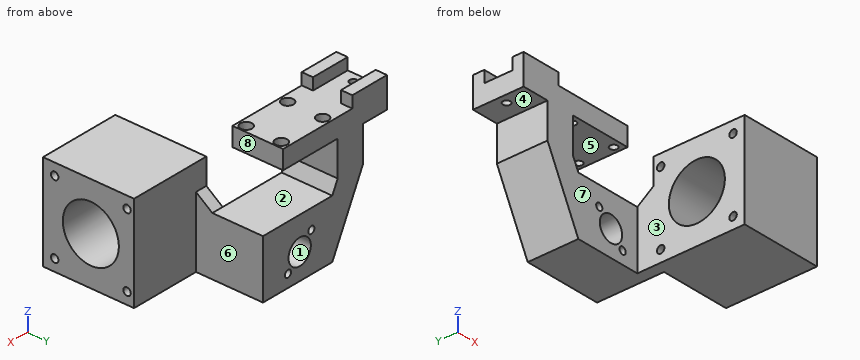
```python
from build123d import *

# Parameters (mm, degrees)
SKICA1_W                 = 50.278910674
SKICA1_H                 = 21.7
SKICA1_R                 = 1.6
P_IDAT_VYSUNUT_M1_DEPTH  = 8
SKICA2_R                 = 2.5
ODEBRAT_VYSUNUT_M1_DEPTH = 4
SKICA3_R                 = 1.6
ODEBRAT_VYSUNUT_M2_DEPTH = 8
SKICA4_W                 = 12.327690559
SKICA4_H                 = 21.7
P_IDAT_VYSUNUT_M2_DEPTH  = 15
SKICA6_R                 = 5.406276896
P_IDAT_VYSUNUT_M3_DEPTH  = 21.7
SKICA7_R                 = 1.5
ODEBRAT_VYSUNUT_M3_DEPTH = 21.7
SKICA9_R                 = 1.6
SKICA9_R_2               = 12
P_IDAT_VYSUNUT_M4_DEPTH  = 5
SKICA10_W                = 41
SKICA10_H                = 39
SKICA10_R                = 12
SKICA10_R_2              = 1.6
P_IDAT_VYSUNUT_M5_DEPTH  = 30
SKICA11_W                = 16.773929501
SKICA11_H                = 4.85
P_IDAT_VYSUNUT_M6_DEPTH  = 5


with BuildPart() as part:
    # Skica1 → Přidat vysunutím1 (new body)
    with BuildSketch(Plane.XY):
        with Locations((-8.927473885, -9.09140889)):
            Rectangle(SKICA1_W, SKICA1_H)
        with Locations((13.311981452, -16.59140889)):
            Circle(SKICA1_R, mode=Mode.SUBTRACT)
        with Locations((-6.688018548, -16.59140889)):
            Circle(SKICA1_R, mode=Mode.SUBTRACT)
        with Locations((-6.688018548, -1.59140889)):
            Circle(SKICA1_R, mode=Mode.SUBTRACT)
        with Locations((13.311981452, -1.59140889)):
            Circle(SKICA1_R, mode=Mode.SUBTRACT)
    extrude(amount=P_IDAT_VYSUNUT_M1_DEPTH)

    # Skica2 → Odebrat vysunutím1 (cut)
    with BuildSketch(Plane.XY.offset(8)):
        with Locations((13.311981452, -16.59140889)):
            Circle(SKICA2_R)
        with Locations((-6.688018548, -16.59140889)):
            Circle(SKICA2_R)
        with Locations((-6.688018548, -1.59140889)):
            Circle(SKICA2_R)
        with Locations((13.311981452, -1.59140889)):
            Circle(SKICA2_R)
    extrude(amount=-ODEBRAT_VYSUNUT_M1_DEPTH, mode=Mode.SUBTRACT)

    # Skica3 → Odebrat vysunutím2 (cut)
    with BuildSketch(Plane.XY.offset(8)):
        with Locations((-30.066929222, -9.09140889)):
            Circle(SKICA3_R)
    extrude(amount=-ODEBRAT_VYSUNUT_M2_DEPTH, mode=Mode.SUBTRACT)

    # Skica4 → Přidat vysunutím2 (add)
    with BuildSketch(Plane(origin=(0, 0, 0), x_dir=(-1, 0, 0), z_dir=(0, 0, -1))):
        with Locations((16.351863828, -9.09140889)):
            Rectangle(SKICA4_W, SKICA4_H)
    extrude(amount=P_IDAT_VYSUNUT_M2_DEPTH)

    # Skica6 → Přidat vysunutím3 (add)
    with BuildSketch(Plane(origin=(0, 1.75859111, 0), x_dir=(1, 0, 0), z_dir=(0, 1, 0))):
        Polygon((-22.515709107, 15), (-10.188018548, 15), (-7.585826442, 20.254970434), (20.97371307, 20.254970434), (20.97371307, 45.15), (4.741864117, 45.15), (-7.585826442, 45.15), align=None)
        with Locations(Location((8.208247023, 34.15, 0), (0, 0, 270))):
            Circle(SKICA6_R, mode=Mode.SUBTRACT)
    extrude(amount=-P_IDAT_VYSUNUT_M3_DEPTH)

    # Skica7 → Odebrat vysunutím3 (cut)
    with BuildSketch(Plane.XZ.offset(19.94140889)):
        with Locations(Location((2.551392773, -28.493145751, 0), (0, 0, 270))):
            Circle(SKICA7_R)
        with Locations(Location((13.865101272, -39.806854249, 0), (0, 0, 270))):
            Circle(SKICA7_R)
    extrude(amount=-ODEBRAT_VYSUNUT_M3_DEPTH, mode=Mode.SUBTRACT)

    # Skica9 → Přidat vysunutím4 (add)
    with BuildSketch(Plane(origin=(20.97371307, 0, 0), x_dir=(0, 0, -1), z_dir=(1, 0, 0))):
        Polygon((45.15, 1.75859111), (20.254970434, 1.75859111), (20.254970434, -19.94140889), (15.15, -26.94140889), (4.15, -26.94140889), (4.15, -65.94140889), (15.15, -65.94140889), (45.15, -65.94140889), (45.15, -19.94140889), align=None)
        with Locations((40.15, -60.94140889)):
            Circle(SKICA9_R, mode=Mode.SUBTRACT)
        with Locations((9.15, -60.94140889)):
            Circle(SKICA9_R, mode=Mode.SUBTRACT)
        with Locations((9.15, -29.94140889)):
            Circle(SKICA9_R, mode=Mode.SUBTRACT)
        with Locations((40.15, -29.94140889)):
            Circle(SKICA9_R, mode=Mode.SUBTRACT)
        with Locations((24.65, -45.44140889)):
            Circle(SKICA9_R_2, mode=Mode.SUBTRACT)
    extrude(amount=P_IDAT_VYSUNUT_M4_DEPTH)

    # Skica10 → Přidat vysunutím5 (add)
    with BuildSketch(Plane(origin=(25.97371307, 0, 0), x_dir=(0, 0, -1), z_dir=(1, 0, 0))):
        with Locations((24.65, -46.44140889)):
            Rectangle(SKICA10_W, SKICA10_H)
        with Locations((24.65, -45.44140889)):
            Circle(SKICA10_R, mode=Mode.SUBTRACT)
        with Locations((40.15, -60.94140889)):
            Circle(SKICA10_R_2, mode=Mode.SUBTRACT)
        with Locations((40.15, -29.94140889)):
            Circle(SKICA10_R_2, mode=Mode.SUBTRACT)
        with Locations((9.15, -29.94140889)):
            Circle(SKICA10_R_2, mode=Mode.SUBTRACT)
        with Locations((9.15, -60.94140889)):
            Circle(SKICA10_R_2, mode=Mode.SUBTRACT)
    extrude(amount=P_IDAT_VYSUNUT_M5_DEPTH)

    # Skica11 → Přidat vysunutím6 (add)
    with BuildSketch(Plane.XY.offset(8)):
        with Locations((-25.679964471, -17.51640889)):
            Rectangle(SKICA11_W, SKICA11_H)
        with Locations((-25.679964471, -0.66640889)):
            Rectangle(SKICA11_W, SKICA11_H)
    extrude(amount=P_IDAT_VYSUNUT_M6_DEPTH)


solid = part.part
```
CAD build for the part. Positions are in the model's coordinates, mm. Face numbers are marked on the shaded views. A direction names the side the tool comes from. Coordinates: 2 decimals unless noted, no trailing zeros. Loops run counter-clockwise (first coordinate to the right, second up) from the corner with the lowest first, then second, coordinate; pieces in that order, holes last. Notation, with made-up numbers: (76.5, 17) - (103.5, 17) arc R8 ccw to (103.5, 30) - close; hole circle Ø5 at (12.25, -2). An arc over 180 degrees is marked (long way). Use CSV: the item, a comma, the result in double quotes. Start each with the question number.
Q1. 3-axis set-ups, long thin cutter, end or side, ignore diameter. For the marked faces 4, 5, 6, 7 and 8: which of +Z, -Z, +X, -X, +Y, -Y reach the whole face in a straight line?
Q2. Cut at C-C, the plane x = 23. List the corners of the cut face in (y, z).
Q3. Cut at A-A, the plane z = 9.5. List the corners of the cut face in (x, y).
Q4. Probe probe 1 along Y at (x, z) = (49.5, -9.15); probe 2 along Z at (x, y) = (14, -3); probe 3 along Z at (x, y) = (9, -4). List the from-to ranges inside material, lowest first. Write a range as from..to.
Q5. Cut at D-D, the plane z = -34.15. List the corners of the cut face in (x, y), then the cut area to 3 significant figures.
Q6. Cut at B-B, the plane y = -54.5. List the corners of the cut face in (x, z).
Q7. Two-plate mould, pull along X, no slides. Class the marked faces 1, 2 and 3: +X half, -X half, draft (parallel to the pull), parting line (faces both ways), or undercut.
Q8. Drop flat-ended pins along their axis: P1, Ø5.5, axis at x = 13, y = -1.5, coming from the +Z side; P2, Ø4, axis at x = -27, z = 10, coming from the -Y side; P3, Ø2.5, axis at x = -7.5, y = -16.5, coming from the +Z side. Give the stop position or say it passes through.
Here are the results:
1,face 4,"-Z, -X, +Y, -Y"
1,face 5,"+X, +Y, -Y"
1,face 6,"+Z, -Z, +X, +Y"
1,face 7,"+Z, -Z, -X, -Y"
1,face 8,"+Z, +X, +Y, -Y"
2,outline,"(-65.94, -45.15) - (1.76, -45.15) - (1.76, -20.25) - (-19.94, -20.25) - (-26.94, -15.15) - (-26.94, -4.15) - (-65.94, -4.15) - close; hole circle Ø3.2 at (-60.94, -40.15); hole circle Ø3.2 at (-60.94, -9.15); hole circle Ø24 at (-45.44, -24.65); hole circle Ø3.2 at (-29.94, -40.15); hole circle Ø3.2 at (-29.94, -9.15)"
3,outline,"(-34.07, -19.94) - (-17.29, -19.94) - (-17.29, -15.09) - (-34.07, -15.09) - close; (-34.07, -3.09) - (-17.29, -3.09) - (-17.29, 1.76) - (-34.07, 1.76) - close"
4,probe 1,"-65.94..-62.54, -59.34..-31.54, -28.34..-26.94"
4,probe 2,"-45.15..-41.3, -38.31..-20.25"
4,probe 3,"-45.15..-39.5, -28.8..-20.25, 0..8"
5,outline,"(-13.03, -19.94) - (2.8, -19.94) - (2.8, 1.76) - (-13.03, 1.76) - close; (13.61, -19.94) - (20.97, -19.94) - (20.97, -38.11) - (55.97, -38.11) - (55.97, -26.94) - (25.97, -26.94) - (25.97, 1.76) - (13.61, 1.76) - close; (20.97, -65.94) - (55.97, -65.94) - (55.97, -52.77) - (20.97, -52.77) - close"
5,area,"1,500 mm2"
6,outline,"(20.97, -45.15) - (55.97, -45.15) - (55.97, -32.52) - (20.97, -32.52) - close; (20.97, -16.78) - (55.97, -16.78) - (55.97, -4.15) - (20.97, -4.15) - close"
7,face 1,"undercut"
7,face 2,"draft"
7,face 3,"-X half"
8,P1,"z = 8"
8,P2,"y = -19.94"
8,P3,"z = 4"
